Verification items for the finished model (mm, model axes). A direction names the side the tool comes from. Give positions to 0.01 mm unless a question says otherwise; leave off trailing zeros. Loops run counter-clockwise (first coordinate to the right, second up) from the corner with the lowest first, then second, coordinate; pieces in that order, holes last. Notation, with made-up numbers: (-13.75, 79.25) - (11.25, 79.25) arc R30 ccw to (11.25, 118.25) - close; hole circle Ø8 at (56, 38). An arc over 180 degrees is marked (long way). One line per item, written item: value. Start each with the question number.
1. Access from +Z, -Z, +X, -X, +Y, -Y to the whole of each face (thin tool, end or side, straight path). Record for faces 3 (the flat face through (245, 760, 0.4)), 4 (the flat face through (272.68, 130.88, 0.01)), 5 (the flat face through (384.867, 1247.025, 0.006)).
2. Sectioned sample at A-A (z = -0.25). Record the cut outline in (x, y) (3 decimals).
3. Mould release check, pull along X, two halves, no side actions. Record for faces 1 (the flat face through (371.109, 129.683, 0.006)), 2 (the flat face through (245, 760, -0.4)): pulls with the +X half, pulls with the -X half, needs draft (parallel to the pull), parting line crosses it, or undercut.
4. Scan lines: L1, parallel to X at y = 1032, z = -0.1; L2, parallel to X at y = 1164, z = 0.35; L3, parallel to X at y = 1396, z = -0.15. Record each from-to range of solid material in increasing order. Write a range as [from, to].
5. Sectioned sample at C-C (x = 212). Record the cut outline in (y, z), plus the area to 3 significant figures.
6. Sectioned sample at B-B (x = 128.5). Record the cut outline in (y, z), plus the area to 3 significant figures.
from build123d import *

# Parameters (mm, degrees)
F0_W     = 50
F0_H     = 173.205
F0_H_2   = 843.832
F0_H_3   = 482.963
F1_DEPTH = 0.4


with BuildPart() as f1:
    # F0 (on Top) → F1 (new body, symmetric)
    with BuildSketch(Plane.XY):
        with Locations((25, 86.6025)):
            Rectangle(F0_W, F0_H)
        with Locations((25, 595.121)):
            Rectangle(F0_W, F0_H_2)
        Polygon((50, 1017.037), (50, 173.205), (248.2458122439, 173.205), (248.2458122439, 1210.1864260022), align=None)
        Polygon((248.2458122439, 173.205), (50, 173.205), (198.6843591829, 87.3620452015), align=None)
        with Locations((25, 1258.5185)):
            Rectangle(F0_W, F0_H_3)
        Polygon((175.0000224798, 1483.543434842), (50, 1017.037), (248.2458122439, 1210.1864260022), align=None)
        Polygon((446.4916244877, 173.205), (248.2458122439, 173.205), (297.8072653048, 87.3620452015), align=None)
        Polygon((248.2458122439, 1210.1864260022), (248.2458122439, 173.205), (446.4916244877, 173.205), (446.4916244877, 1017.037), align=None)
        Polygon((321.4916020079, 1483.543434842), (248.2458122439, 1210.1864260022), (446.4916244877, 1017.037), align=None)
        with Locations((471.4916244877, 595.121)):
            Rectangle(F0_W, F0_H_2)
        with Locations((471.4916244877, 86.6025)):
            Rectangle(F0_W, F0_H)
        with Locations((471.4916244877, 1258.5185)):
            Rectangle(F0_W, F0_H_3)
    extrude(amount=F1_DEPTH, both=True)


solid = f1.part
Results are:
1. face 3: +Z, +X, -X, +Y, -Y
1. face 4: +Z, -Z, -Y
1. face 5: +Z, -Z, +Y
2. outline: (0, 0) - (50, 0) - (50, 173.205) - (198.684, 87.362) - (248.246, 173.205) - (297.807, 87.362) - (446.492, 173.205) - (446.492, 0) - (496.492, 0) - (496.492, 1500) - (446.492, 1500) - (446.492, 1017.037) - (321.492, 1483.543) - (248.246, 1210.186) - (175, 1483.543) - (50, 1017.037) - (50, 1500) - (0, 1500) - close
3. face 1: undercut
3. face 2: needs draft
4. L1: x = [0, 50], [54.01, 442.48], [446.49, 496.49]
4. L2: x = [0, 50], [89.38, 407.11], [446.49, 496.49]
4. L3: x = [0, 50], [151.54, 198.46], [298.03, 344.95], [446.49, 496.49]
5. outline: (110.43, -0.4) - (1345.46, -0.4) - (1345.46, 0.4) - (110.43, 0.4) - close
5. area: 988 mm^2
6. outline: (127.88, -0.4) - (1310, -0.4) - (1310, 0.4) - (127.88, 0.4) - close
6. area: 946 mm^2
